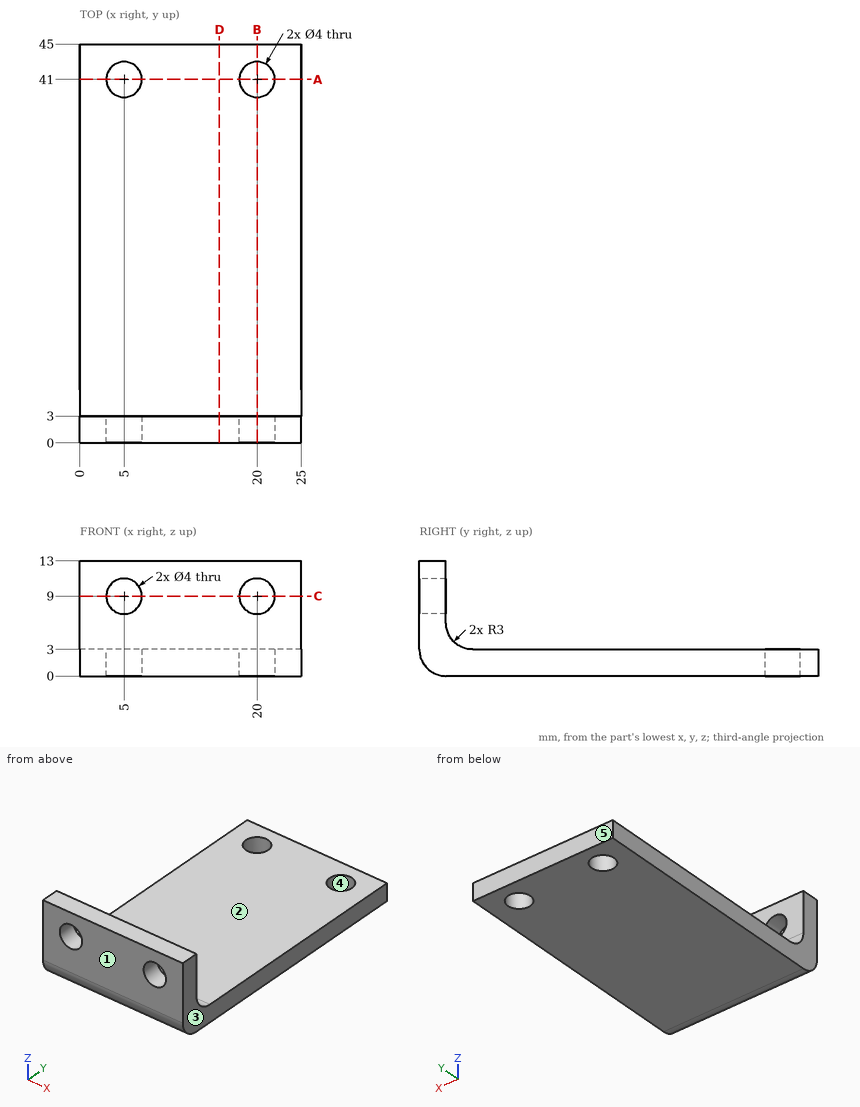
For this review, use the dimensioned drawing (mm, ordinates from the lowest corner) and the shaded views. A direction names the side the tool comes from. Coordinates: 2 decimals unless noted, no trailing zeros. Order: outer loops, then holes, each group sorted by start corner. A loop starts at its lowest first (then second) coordinate and runs counter-clockwise, first axis right, second up. Notation, with made-up numbers: M 61.5,-7 L 80.5,-7 A25 cw 80.5,28 Z; hole C -10.75,19.25 d8. An arc over 180 degrees is marked long. Answer as a JSON object with one key per item and string values. Group by question number.
1) Tool access review of the marked faces 1 and 2: name each direction out of +Z, -Z, +X, -X, +Y, -Y from which nothing blocks a thin tool from reaching the whole face with its end or side.
2) Add section D-D, the plane x = 15.75. Write out the cut boundary in (y, z), then the cut area to 3 significant figures.
3) Add section A-A, the plane y = 41. Write out the cut boundary in (x, z), then the cut area to 3 significant figures.
4) For pin 1 (1 mm diameter, centred on x = 13, y = 31.5, fed in from -Z); pin 2 (3 mm diameter, centred on x = 20, y = 33.5, fed in from +Z); pin 3 (3 mm diameter, centred on x = 5, z = 9, fed in from +Y); pin 4 (5.5 mm diameter, centred on x = 6.5, z = 8, fed in from +Y), all flat-tipped, find the tip position at first contact; note any pin that passes through.
5) Mouldability with a two-part tool opening along Y and no side actions: class the marked faces 3, 4 and 5 as pulls with the +Y half, pulls with the -Y half, needs draft (parallel to the pull), parting line crosses it, or undercut.
6) Wall thickness on L1, parallel to Y at x = 8, z = 5.75; L2, parallel to Z at x = 18.25, y = 10; L3, parallel to Y at x = 20, z = 1.35: over which ranges is each line inside the solid? List them lowest first.
7) Add section B-B, the plane x = 20. Write out the cut boundary in (y, z), then the cut area to 3 significant figures.
Computed values:
{
 "1": {"face 1": "+Z, -Z, +X, -X, -Y", "face 2": "+Z, +X, -X, +Y"},
 "2": {"outline": "M 0,3 A3 ccw 3,0 L 45,0 L 45,3 L 6,3 A3 cw 3,6 L 3,13 L 0,13 Z", "area": "165 mm^2"},
 "3": {"outline": "M 0,0 L 3,0 L 3,3 L 0,3 Z; M 7,0 L 18,0 L 18,3 L 7,3 Z; M 22,0 L 25,0 L 25,3 L 22,3 Z", "area": "51.0 mm^2"},
 "4": {"pin 1": "stops at z = 0", "pin 2": "stops at z = 3", "pin 3": "passes through", "pin 4": "stops at y = 3.1"},
 "5": {"face 3": "needs draft", "face 4": "undercut", "face 5": "pulls with the +Y half"},
 "6": {"L1": "y = 0 to 3.01", "L2": "z = 0 to 3", "L3": "y = 0.49 to 39, 43 to 45"},
 "7": {"outline": "M 0,3 A3 ccw 3,0 L 39,0 L 39,3 L 6,3 A3 cw 3,6 L 3,7 L 0,7 Z; M 0,11 L 3,11 L 3,13 L 0,13 Z; M 43,0 L 45,0 L 45,3 L 43,3 Z", "area": "141 mm^2"}
}
